from build123d import *

# Parameters (mm, degrees)
SKETCH_6_R         = 6
EXTRUDE_4_DEPTH    = 4
FILLET_2_R         = 2
FILLET_6_R         = 2
FILLET_12_R        = 2
FILLET_16_R        = 2
HOLE_WIZARD_M4_1_D = 3.3


with BuildPart() as part:
    # 草图6 → 凸台-拉伸4 (new body)
    with BuildSketch(Plane.XY):
        Polygon((-15, -22.5), (-15, -30), (-7.5, -30), (7.5, -30), (15, -30), (15, -22.5), (15, 22.5), (15, 30), (7.5, 30), (-7.5, 30), (-15, 30), (-15, 22.5), align=None)
        Circle(SKETCH_6_R, mode=Mode.SUBTRACT)
    extrude(amount=EXTRUDE_4_DEPTH)

    # 圆角2
    fillet_2_edges = [part.edges().sort_by_distance(p)[0] for p in [
        (15, 30, 2),
    ]]
    fillet(fillet_2_edges, radius=FILLET_2_R)

    # 圆角6
    fillet_6_edges = [part.edges().sort_by_distance(p)[0] for p in [
        (15, -30, 2),
    ]]
    fillet(fillet_6_edges, radius=FILLET_6_R)

    # 圆角12
    fillet_12_edges = [part.edges().sort_by_distance(p)[0] for p in [
        (-15, 30, 2),
    ]]
    fillet(fillet_12_edges, radius=FILLET_12_R)

    # 圆角16
    fillet_16_edges = [part.edges().sort_by_distance(p)[0] for p in [
        (-15, -30, 2),
    ]]
    fillet(fillet_16_edges, radius=FILLET_16_R)

    # M4 螺纹孔1 (through all)
    with Locations(Plane.XY.offset(4)):
        with Locations((-11.25, 26.25), (11.25, 26.25), (11.25, -26.25), (-11.25, -26.25)):
            Hole(HOLE_WIZARD_M4_1_D / 2)


solid = part.part
Verification items for the finished model (mm, model axes). Coordinates: 2 decimals unless noted, no trailing zeros. Write each loop counter-clockwise with the first axis right and the second up, starting at its lowest first coordinate (ties: lowest second). Pieces come first, ordered by that corner, then holes. Notation, with made-up numbers: M -25,58 L 28,58 A13 ccw 28,81 Z; hole C 76.25,20 d3. An arc over 180 degrees is marked long. One line per question, with ' | ' between items.
1) Sectioned sample at C-C on z = 1.1. Record the cut outline in (x, y).
Solutions:
outline: M -15,-28 A2 ccw -13,-30 L 13,-30 A2 ccw 15,-28 L 15,28 A2 ccw 13,30 L -13,30 A2 ccw -15,28 Z; hole C -11.25,-26.25 d3.3; hole C -11.25,26.25 d3.3; hole C 0,0 d12; hole C 11.25,-26.25 d3.3; hole C 11.25,26.25 d3.3
2) Depth check by flat-ended pin: pin 1 Ø4.5 at (x, y) = (-11.25, -26.25) entering from -Z. Enter the tip coordinate at first touch or a pass-through.
Solutions:
pin 1: z = 0
3) Sectioned sample at B-B on y = 0. Record the cut outline in (x, z).
Solutions:
outline: M -15,0 L -6,0 L -6,4 L -15,4 Z; M 6,0 L 15,0 L 15,4 L 6,4 Z
4) Sectioned sample at A-A on x = -11.25. Record the cut outline in (y, z), then the cut area to 3 significant figures.
Solutions:
outline: M -30,0 L -27.9,0 L -27.9,4 L -30,4 Z; M -24.6,0 L 24.6,0 L 24.6,4 L -24.6,4 Z; M 27.9,0 L 30,0 L 30,4 L 27.9,4 Z | area: 214 mm^2
5) Material ranges on L1, parallel to Y at x = -11.25, z = 3.1; L2, parallel to Y at x = 0, z = 1.6; L3, parallel to Y at x = -10.25, z = 2.75, recorded low to high.
Solutions:
L1: -30 to -27.9, -24.6 to 24.6, 27.9 to 30 | L2: -30 to -6, 6 to 30 | L3: -30 to -27.56, -24.94 to 24.94, 27.56 to 30
